```python
from build123d import *

# Parameters (mm, degrees)
SKETCH2_W           = 177.8
SKETCH2_H           = 50.8
SKETCH2_R           = 2.54
BOSS_EXTRUDE1_DEPTH = 3.175


with BuildPart() as part:
    # Sketch2 → Boss-Extrude1 (new body)
    with BuildSketch(Plane(origin=(0, 0, 0), x_dir=(1, 0, 0), z_dir=(0, 1, 0))):
        Rectangle(SKETCH2_W, SKETCH2_H)
        with Locations(Location((-76.2, -12.7, 0), (0, 0, 270))):
            Circle(SKETCH2_R, mode=Mode.SUBTRACT)
        with Locations(Location((-76.2, 12.7, 0), (0, 0, 270))):
            Circle(SKETCH2_R, mode=Mode.SUBTRACT)
        with Locations(Location((-50.8, -12.7, 0), (0, 0, 270))):
            Circle(SKETCH2_R, mode=Mode.SUBTRACT)
        with Locations(Location((-50.8, 12.7, 0), (0, 0, 270))):
            Circle(SKETCH2_R, mode=Mode.SUBTRACT)
        with Locations(Location((-25.4, -12.7, 0), (0, 0, 270))):
            Circle(SKETCH2_R, mode=Mode.SUBTRACT)
        with Locations(Location((-25.4, 12.7, 0), (0, 0, 270))):
            Circle(SKETCH2_R, mode=Mode.SUBTRACT)
        with Locations(Location((0, -12.7, 0), (0, 0, 270))):
            Circle(SKETCH2_R, mode=Mode.SUBTRACT)
        with Locations(Location((0, 12.7, 0), (0, 0, 270))):
            Circle(SKETCH2_R, mode=Mode.SUBTRACT)
        with Locations(Location((25.4, -12.7, 0), (0, 0, 270))):
            Circle(SKETCH2_R, mode=Mode.SUBTRACT)
        with Locations(Location((25.4, 12.7, 0), (0, 0, 270))):
            Circle(SKETCH2_R, mode=Mode.SUBTRACT)
        with Locations(Location((50.8, -12.7, 0), (0, 0, 270))):
            Circle(SKETCH2_R, mode=Mode.SUBTRACT)
        with Locations(Location((50.8, 12.7, 0), (0, 0, 270))):
            Circle(SKETCH2_R, mode=Mode.SUBTRACT)
        with Locations(Location((76.2, -12.7, 0), (0, 0, 270))):
            Circle(SKETCH2_R, mode=Mode.SUBTRACT)
        with Locations(Location((76.2, 12.7, 0), (0, 0, 270))):
            Circle(SKETCH2_R, mode=Mode.SUBTRACT)
    extrude(amount=BOSS_EXTRUDE1_DEPTH)


solid = part.part
```
Could you check a few things on this model? Use its own coordinates, in mm. Round coordinates to 2 decimals unless told otherwise and drop trailing zeros. Loops run counter-clockwise (first coordinate to the right, second up) from the corner with the lowest first, then second, coordinate; pieces in that order, holes last. Notation, with made-up numbers: (-20, 57) - (14, 57) arc R12 ccw to (14, 69) - close; hole circle Ø11 at (49.5, -25). An arc over 180 degrees is marked (long way). Answer as CSV lines item,"result".
1. I want a section at B-B on x = 0. List the corners of the cut face in (y, z) for me (3 decimals).
Filled in:
outline,"(0, -25.4) - (3.175, -25.4) - (3.175, -15.24) - (0, -15.24) - close; (0, -10.16) - (3.175, -10.16) - (3.175, 10.16) - (0, 10.16) - close; (0, 15.24) - (3.175, 15.24) - (3.175, 25.4) - (0, 25.4) - close"
2. We'd pull the mould along X, two halves only. Please class faces 1 (the face through (88.9, 2, 0)), 2 (the face through (27.92, 1.57, 12.37)), 3 (the face through (-1, 2, -25.4)): +X half, -X half, draft (parallel to the pull), parting line (faces both ways), or undercut.
Filled in:
face 1,"+X half"
face 2,"undercut"
face 3,"draft"
3. For pin 1 Ø4.5 at (x, z) = (0, -12.7) entering from -Y, with a flat end and sliding along its axis, tell me the tip position at first contact or that it passes through.
Filled in:
pin 1,"passes through"
4. I want a section at A-A on z = -12.7. Count the separate pieces of the cut face and the enclosed holes in it, then the cut area to 3 significant figures.
Filled in:
separate pieces,"8"
enclosed holes,"0"
area,"452 mm^2"
